from build123d import *

# Parameters (mm, degrees)
F0_R     = 10
F0_W     = 40
F0_H     = 20
F1_DEPTH = 30


with BuildPart() as f1:
    # F0 (on Front) → F1 (new body)
    with BuildSketch(Plane.XZ):
        with BuildLine():
            Line((75.732799, 90.009839), (-24.267201, 90.009839))
            ThreePointArc((-24.267201, 90.009839), (-31.338269, 87.080907), (-34.267201, 80.009839))
            ThreePointArc((-34.267201, 80.009839), (-37.196133, 72.938771), (-44.267201, 70.009839))
            Line((-44.267201, 70.009839), (-74.267201, 70.009839))
            ThreePointArc((-74.267201, 70.009839), (-81.338269, 67.080907), (-84.267201, 60.009839))
            Line((-84.267201, 60.009839), (-84.267201, -19.990161))
            ThreePointArc((-84.267201, -19.990161), (-81.338269, -27.061229), (-74.267201, -29.990161))
            Line((-74.267201, -29.990161), (-44.267201, -29.990161))
            ThreePointArc((-44.267201, -29.990161), (-37.196133, -32.919093), (-34.267201, -39.990161))
            ThreePointArc((-34.267201, -39.990161), (-31.338269, -47.061229), (-24.267201, -49.990161))
            Line((-24.267201, -49.990161), (75.732799, -49.990161))
            ThreePointArc((75.732799, -49.990161), (82.803867, -47.061229), (85.732799, -39.990161))
            ThreePointArc((85.732799, -39.990161), (88.661731, -32.919093), (95.732799, -29.990161))
            Line((95.732799, -29.990161), (105.732799, -29.990161))
            ThreePointArc((105.732799, -29.990161), (112.803867, -27.061229), (115.732799, -19.990161))
            Line((115.732799, -19.990161), (115.732799, 50.099277))
            ThreePointArc((115.732799, 50.099277), (112.803867, 57.170345), (105.732799, 60.099277))
            Line((105.732799, 60.099277), (95.732799, 60.099277))
            ThreePointArc((95.732799, 60.099277), (88.661731, 63.028209), (85.732799, 70.099277))
            Line((85.732799, 70.099277), (85.732799, 80.009839))
            ThreePointArc((85.732799, 80.009839), (82.803867, 87.080907), (75.732799, 90.009839))
        make_face()
        with BuildLine():
            Line((-44.267201, -20), (-74.267201, -20))
            Line((-74.267201, -20), (-74.267201, 0))
            Line((-74.267201, 0), (-34.267201, 0))
            Line((-34.267201, 0), (-34.267201, -10))
            ThreePointArc((-34.267201, -10), (-37.196133, -17.071068), (-44.267201, -20))
        make_face(mode=Mode.SUBTRACT)
        with BuildLine():
            ThreePointArc((70.956033, -19.990161), (68.0271, -27.061229), (60.956033, -29.990161))
            Line((60.956033, -29.990161), (0.956033, -29.990161))
            ThreePointArc((0.956033, -29.990161), (-6.115035, -27.061229), (-9.043967, -19.990161))
            Line((-9.043967, -19.990161), (-9.043967, 20.009839))
            Line((-9.043967, 20.009839), (70.956033, 20.009839))
            Line((70.956033, 20.009839), (70.956033, -19.990161))
        make_face(mode=Mode.SUBTRACT)
        with Locations((95.693012, -14.23213)):
            Circle(F0_R, mode=Mode.SUBTRACT)
        with Locations((94.65915, 15.750051)):
            Circle(F0_R, mode=Mode.SUBTRACT)
        with Locations((-54.267201, 20.009839)):
            Rectangle(F0_W, F0_H, mode=Mode.SUBTRACT)
        with BuildLine():
            Line((-74.267201, 40.019678), (-74.267201, 60.019678))
            Line((-74.267201, 60.019678), (-44.267201, 60.019678))
            ThreePointArc((-44.267201, 60.019678), (-37.196133, 57.090745), (-34.267201, 50.019678))
            Line((-34.267201, 50.019678), (-34.267201, 40.019678))
            Line((-34.267201, 40.019678), (-74.267201, 40.019678))
        make_face(mode=Mode.SUBTRACT)
        with Locations((94.02099, 45.743262)):
            Circle(F0_R, mode=Mode.SUBTRACT)
        with BuildLine():
            ThreePointArc((-9.043967, 60.009839), (-6.115035, 67.080907), (0.956033, 70.009839))
            Line((0.956033, 70.009839), (60.956033, 70.009839))
            ThreePointArc((60.956033, 70.009839), (68.0271, 67.080907), (70.956033, 60.009839))
            Line((70.956033, 60.009839), (70.956033, 45.009839))
            Line((70.956033, 45.009839), (-9.043967, 45.009839))
            Line((-9.043967, 45.009839), (-9.043967, 60.009839))
        make_face(mode=Mode.SUBTRACT)
    extrude(amount=F1_DEPTH)


solid = f1.part
The listing builds one solid part. Answer for the finished solid, in the listing's coordinates (mm). A direction names the side the tool comes from. Coordinates: 2 decimals unless noted, no trailing zeros. Write each loop counter-clockwise with the first axis right and the second up, starting at its lowest first coordinate (ties: lowest second). Pieces come first, ordered by that corner, then holes. Notation, with made-up numbers: (10.5, -13) - (28.5, -13) arc R20 cw to (28.5, 3) - close; hole circle Ø6 at (59, -15.5). An arc over 180 degrees is marked (long way). Return JSON: item names as keys, results as strings.
1. Which of the six approach directions +Z, -Z, +X, -X, +Y, -Y give full straight-line access (tool end or side, diameter ignored) to faces 1 (the face through (-59, -15, -29.99)), 2 (the face through (-34.267, -15, 20)), 3 (the face through (14, -30, 21)), 4 (the face through (85.733, -15, 75))?
Final values:
{"face 1": "-Z, -X, +Y, -Y", "face 2": "+Y, -Y", "face 3": "+Z, -Z, +X, -X, -Y", "face 4": "+Z, +X, +Y, -Y"}
2. Consider line 1 along Z through (x, y) = (58, -5.5); line 2 along Z through (x, y) = (-49, -3); line 3 along X through (y, z) = (-28.5, 26). Determine where each line is inside the solid, lowest interval first.
Final values:
{"line 1": "-49.99 to -29.99, 20.01 to 45.01, 70.01 to 90.01", "line 2": "-29.99 to -20, 0 to 10.01, 30.01 to 40.02, 60.02 to 70.01", "line 3": "-84.27 to -74.27, -34.27 to 115.73"}
3. The part is cut by section D-D on x = -40. Determine the outline of the cut face in (y, z), then the cut area to 3 significant figures.
Final values:
{"outline": "(-30, -30.95) - (0, -30.95) - (0, -19.04) - (-30, -19.04) - close; (-30, 0) - (0, 0) - (0, 10.01) - (-30, 10.01) - close; (-30, 30.01) - (0, 30.01) - (0, 40.02) - (-30, 40.02) - close; (-30, 59.06) - (0, 59.06) - (0, 70.97) - (-30, 70.97) - close", "area": "1,310 mm^2"}
4. Each of these flat-tipped pins is pushed along its axis until it touches: pin 1 Ø15 at (x, y) = (-57, -21.5) entering from -Z; pin 2 Ø6 at (y, z) = (-12.5, 53) entering from +X; pin 3 Ø3 at (x, z) = (89, 68.5) entering from -Y; pin 4 Ø15 at (x, y) = (-62, -11.5) entering from +Z. Where does it stop, or does it pass through?
Final values:
{"pin 1": "z = -29.99", "pin 2": "x = 115.73", "pin 3": "through", "pin 4": "z = 70.01"}
5. The part is cut by section B-B on x = 91. Determine the outline of the cut face in (y, z), then the cut area to 3 significant figures.
Final values:
{"outline": "(-30, -31.18) - (0, -31.18) - (0, -23.06) - (-30, -23.06) - close; (-30, -5.4) - (0, -5.4) - (0, 6.44) - (-30, 6.44) - close; (-30, 25.06) - (0, 25.06) - (0, 36.21) - (-30, 36.21) - close; (-30, 55.28) - (0, 55.28) - (0, 61.29) - (-30, 61.29) - close", "area": "1,110 mm^2"}
6. For a pull along X with two mould halves and no side action, classify faces 5 (the face through (-84.267, -15, 21)), 6 (the face through (-9.044, -15, 0)), 7 (the face through (82.881, -14.79, 87.003)) as +X half, -X half, draft (parallel to the pull), parting line (faces both ways), or undercut.
Final values:
{"face 5": "-X half", "face 6": "undercut", "face 7": "+X half"}
7. The part is cut by section C-C on z = 22. Determine the outline of the cut face in (x, y).
Final values:
{"outline": "(-84.27, -30) - (-74.27, -30) - (-74.27, 0) - (-84.27, 0) - close; (-34.27, -30) - (86.85, -30) - (86.85, 0) - (-34.27, 0) - close; (102.47, -30) - (115.73, -30) - (115.73, 0) - (102.47, 0) - close"}
8. The part is cut by section A-A on z = 2.5. Determine the outline of the cut face in (x, y), then the cut area to 3 significant figures.
Final values:
{"outline": "(-84.27, -30) - (-9.04, -30) - (-9.04, 0) - (-84.27, 0) - close; (70.96, -30) - (115.73, -30) - (115.73, 0) - (70.96, 0) - close", "area": "3,600 mm^2"}
